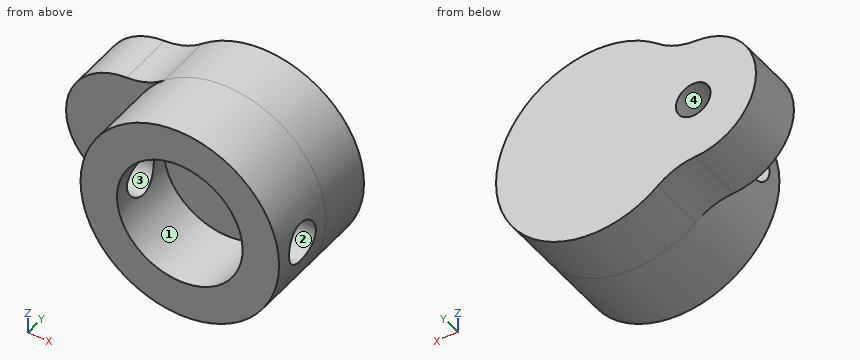
from build123d import *

# Parameters (mm, degrees)
SKETCH1_R               = 10.033
SKETCH1_R_2             = 6.35
BOSS_EXTRUDE1_DEPTH     = 7.1628
CUT_EXTRUDE1_DEPTH      = 16.894271982
CUT_EXTRUDE1_DEPTH_BACK = 16.894271982
SKETCH2_R               = 2.05105
SKETCH3_R               = 1.75
BOSS_EXTRUDE2_DEPTH     = 5.7912


with BuildPart() as part:
    # Sketch1 → Boss-Extrude1 (new body)
    with BuildSketch(Plane(origin=(0, 0, 0), x_dir=(1, 0, 0), z_dir=(0, 1, 0))):
        with Locations(Location((0, 0, 0), (0, 0, 270))):
            Circle(SKETCH1_R)
        with Locations(Location((0, 0, 0), (0, 0, 270))):
            Circle(SKETCH1_R_2, mode=Mode.SUBTRACT)
    extrude(amount=BOSS_EXTRUDE1_DEPTH)

    # Sketch2 → Cut-Extrude1 (cut, two sides: drawn at the far end of the back side and taken through both)
    with BuildSketch(Plane(origin=(0, 0, 0), x_dir=(0, 0, -1), z_dir=(1, 0, 0)).offset(-CUT_EXTRUDE1_DEPTH_BACK)):
        with Locations((0, 3.5687)):
            Circle(SKETCH2_R)
    extrude(amount=CUT_EXTRUDE1_DEPTH + CUT_EXTRUDE1_DEPTH_BACK, mode=Mode.SUBTRACT)

    # Sketch3 → Boss-Extrude2 (add)
    with BuildSketch(Plane(origin=(0, 7.1628, 0), x_dir=(1, 0, 0), z_dir=(0, 1, 0))):
        with BuildLine():
            ThreePointArc((-6.34436033, -7.772398665), (10.033, 0), (-6.34436033, 7.772398665))
            ThreePointArc((-6.34436033, 7.772398665), (-8.120246687, 6.749669096), (-10.12938913, 6.345819163))
            ThreePointArc((-10.12938913, 6.345819163), (-16.249, 0), (-10.12938913, -6.345819163))
            ThreePointArc((-10.12938913, -6.345819163), (-8.120246687, -6.749669096), (-6.34436033, -7.772398665))
        make_face()
        with Locations(Location((-9.899, 0, 0), (0, 0, 89.352367696))):
            Circle(SKETCH3_R, mode=Mode.SUBTRACT)
    extrude(amount=BOSS_EXTRUDE2_DEPTH)


solid = part.part
Work out the finished part from the listing and answer in its coordinate system (mm). Face numbers are marked on the shaded views. A direction names the side the tool comes from. Give positions to 0.01 mm unless a question says otherwise; leave off trailing zeros. Loops run counter-clockwise (first coordinate to the right, second up) from the corner with the lowest first, then second, coordinate; pieces in that order, holes last. Notation, with made-up numbers: (13, -31.5) - (60, -31.5) arc R15 ccw to (60, -3.5) - close; hole circle Ø10 at (83.5, 3.25). An arc over 180 degrees is marked (long way). Answer in a Markdown table with one row per item. Add a question column.
Q1. A tool of negligible diameter and unlimited length cuts with its end or side. For the marked faces 1 and 2, from which of +Z, -Z, +X, -X, +Y, -Y can it reach the whole face along a straight path? Write none if from no direction.
Q2. The part is cut by section D-D (x = -7). Determine the outline of the cut face in (y, z).
Q3. Each of these flat-tipped pins is pushed along its axis until it touches: P1, Ø2, axis at y = 6, z = 6.5, coming from the +X side; P2, Ø6, axis at y = 10, z = -5, coming from the -X side; P3, Ø1.5, axis at x = 1.5, y = 11, coming from the +Z side. Where does it stop, or does it pass through?
Q4. The part is cut by section C-C (y = 4). Determine the outline of the cut face in (x, z), and give its area (3 significant figures).
Q5. Consider line 1 along Y through (x, z) = (-8.1, 0); line 2 along Y through (x, z) = (-9, 0); line 3 along Y through (x, z) = (-6, -0.25). Determine where each line is inside the solid, lowest interval first.
Q6. The part is cut by section B-B (x = 0). Determine the outline of the cut face in (y, z).
Q7. The part is cut by section A-A (z = 0). Determine the outline of the cut face in (x, y), and give its area (3 significant figures).
Q8. Determine the mould class of the marked faces 3 and 4 for opening direction X: released by +X, released by -X, zero draft, split by the parting line, or undercut.
Solution:
| question | item | result |
|---|---|---|
| 1 | face 1 | -Y |
| 1 | face 2 | +X, -X |
| 2 | outline | (0, -7.19) - (7.16, -7.19) - (7.16, -7.3) - (12.95, -7.3) - (12.95, 7.3) - (7.16, 7.3) - (7.16, 7.19) - (0, 7.19) - close; hole circle Ø4.1 at (3.57, 0) |
| 3 | P1 | stops at x = 8.39 |
| 3 | P2 | stops at x = -15.93 |
| 3 | P3 | stops at z = 10 |
| 4 | outline | (-9.83, -2.01) arc R10.03 ccw to (9.83, -2.01) - (6.03, -2.01) arc R6.35 cw to (-6.03, -2.01) - close; (-9.83, 2.01) - (-6.03, 2.01) arc R6.35 cw to (6.03, 2.01) - (9.83, 2.01) arc R10.03 ccw to start |
| 4 | area | 160 mm² |
| 5 | line 1 | y = 0 to 1.52, 5.62 to 12.95 |
| 5 | line 2 | y = 0 to 1.52, 5.62 to 7.16 |
| 5 | line 3 | y = 7.16 to 12.95 |
| 6 | outline | (0, -10.03) - (12.95, -10.03) - (12.95, 10.03) - (0, 10.03) - (0, 6.35) - (7.16, 6.35) - (7.16, -6.35) - (0, -6.35) - close |
| 7 | outline | (-16.25, 7.16) - (-11.65, 7.16) - (-11.65, 12.95) - (-16.25, 12.95) - close; (-10.03, 0) - (-6.35, 0) - (-6.35, 1.52) - (-10.03, 1.52) - close; (-10.03, 5.62) - (-6.35, 5.62) - (-6.35, 7.16) - (6.35, 7.16) - (6.35, 5.62) - (10.03, 5.62) - (10.03, 12.95) - (-8.15, 12.95) - (-8.15, 7.16) - (-10.03, 7.16) - close; (6.35, 0) - (10.03, 0) - (10.03, 1.52) - (6.35, 1.52) - close |
| 7 | area | 154 mm² |
| 8 | face 3 | zero draft |
| 8 | face 4 | undercut |
